The drawing under review shows one solid part. Ordinate dimensions are in mm from its lowest x, y, z. Coordinates: 2 decimals unless noted, no trailing zeros. Write each loop counter-clockwise with the first axis right and the second up, starting at its lowest first coordinate (ties: lowest second). Pieces come first, ordered by that corner, then holes. Notation, with made-up numbers: (8, 39) -> (15, 39) arc R9 ccw to (15, 52) -> close; hole circle Ø9 at (59.25, 72). An arc over 180 degrees is marked (long way). One line per question, with ' | ' between items. Start each with the question number.
Q1. Wall thickness on probe 1 along Y at (x, z) = (113, 60.75): over which ranges is the line inside the solid? List them lowest first.
Q2. For P1, Ø5, axis at x = 56.5, z = 40.5, coming from the -Y side; P2, Ø5, axis at x = 7, y = 7, coming from the +Z side, all flat-tipped, find the tip position at first contact; note any pin that passes through.
Q3. Add section A-A on x = 113. State the section outline as (y, z) points, and give its area (3 significant figures).
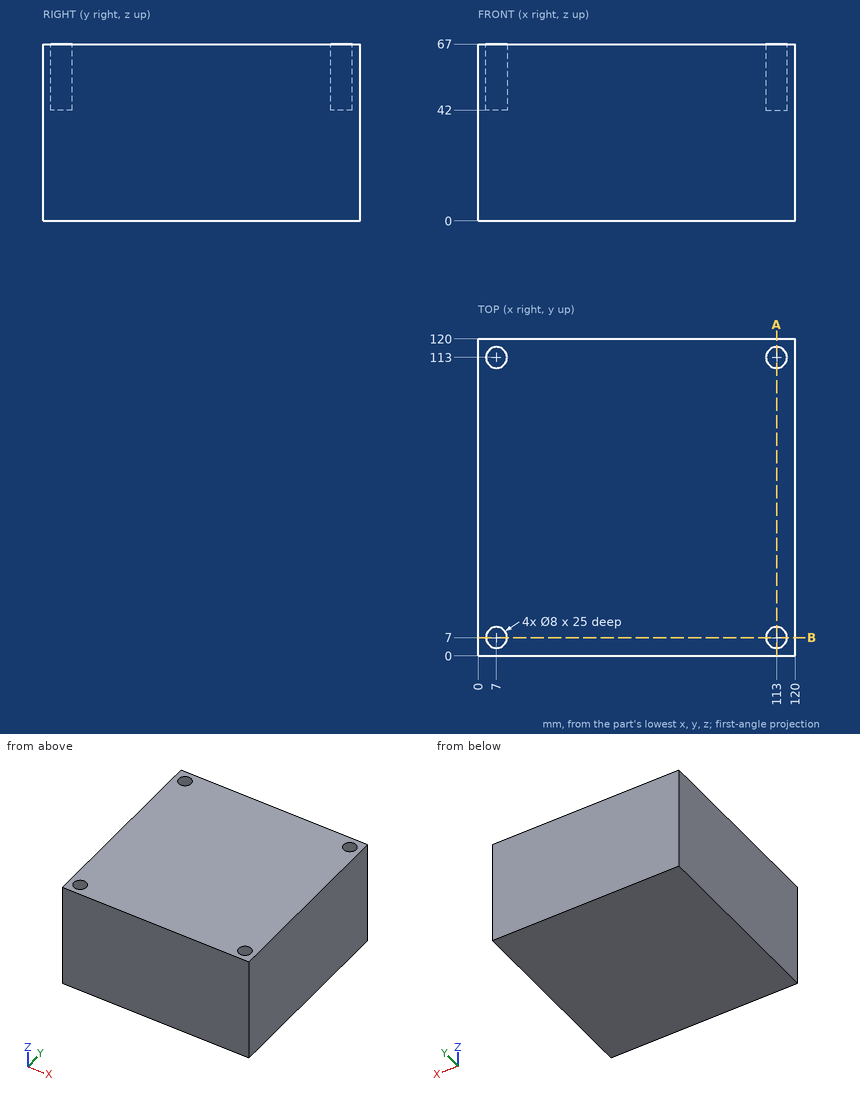
Output values:
1) probe 1: y = 0 to 3, 11 to 109, 117 to 120
2) P1: stops at y = 0 | P2: stops at z = 42
3) outline: (0, 0) -> (120, 0) -> (120, 67) -> (117, 67) -> (117, 42) -> (109, 42) -> (109, 67) -> (11, 67) -> (11, 42) -> (3, 42) -> (3, 67) -> (0, 67) -> close | area: 7,640 mm2
